Design review of the part shown in the three views and the two pictorial views. Dimensions are in mm from the part's minimum x, y and z. Round coordinates to 2 decimals unless told otherwise and drop trailing zeros. Write each loop counter-clockwise with the first axis right and the second up, starting at its lowest first coordinate (ties: lowest second). Pieces come first, ordered by that corner, then holes. Notation, with made-up numbers: (63, 71) - (70, 71) arc R21 ccw to (70, 87) - close; hole circle Ø11 at (58.5, 71). An arc over 180 degrees is marked (long way). One line per item, written item: value. Start each with the question number.
Q1. Add section D-D on y = 37.5. Write out the cut boundary in (x, z), and give its area (3 significant figures).
Q2. For probe 1 along Z at (x, y) = (15.5, 21); probe 2 along X at (y, z) = (3, 3.5), list the stretches that pass through material, from the lowest coordinate up.
Q3. Add section B-B on x = 27.5. Write out the cut boundary in (y, z), and give its area (3 significant figures).
Q4. Add section A-A on y = 22. Write out the cut boundary in (x, z), and give its area (3 significant figures).
Q5. Mouldability with a two-part tool opening along Z and no side actions: class the marked faces 1, 2 and 3 as +Z half, -Z half, draft (parallel to the pull), parting line (faces both ways), or undercut.
Q6. Add section C-C on x = 17. Write out the cut boundary in (y, z), and give its area (3 significant figures).
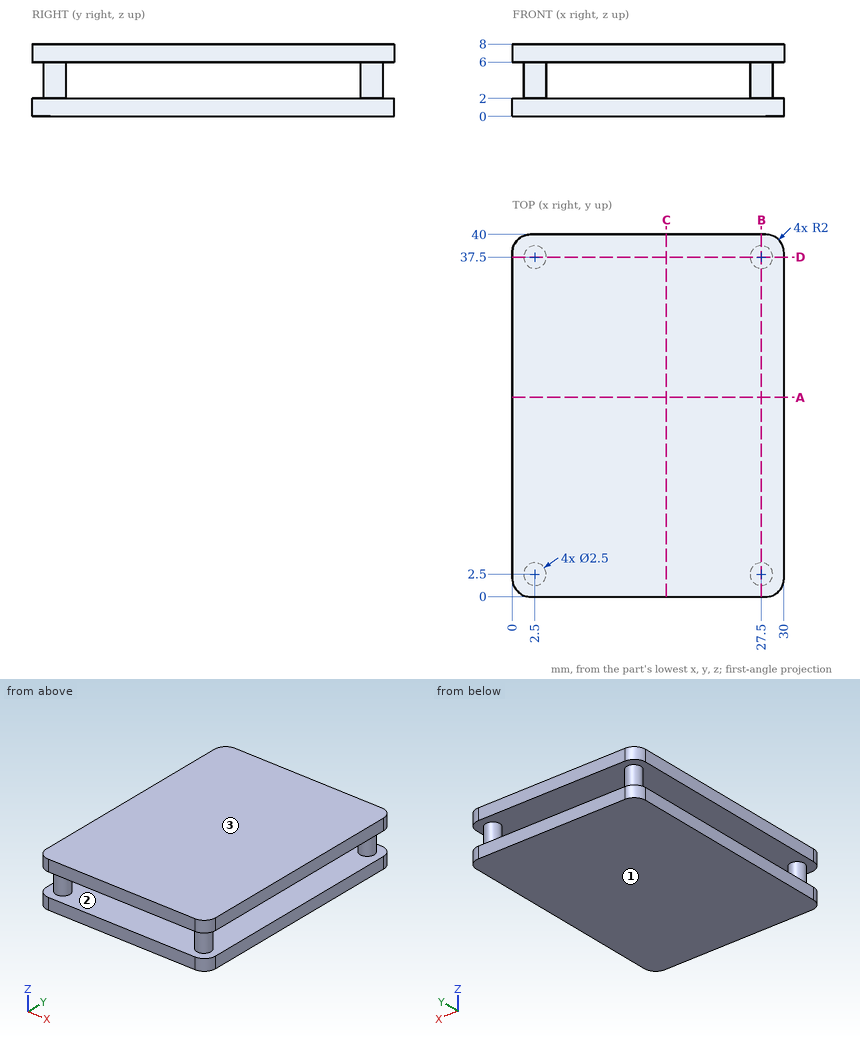
Result set:
1. outline: (0, 0) - (30, 0) - (30, 2) - (28.75, 2) - (28.75, 6) - (30, 6) - (30, 8) - (0, 8) - (0, 6) - (1.25, 6) - (1.25, 2) - (0, 2) - close; hole (3.75, 2) - (26.25, 2) - (26.25, 6) - (3.75, 6) - close
1. area: 140 mm^2
2. probe 1: z = 0 to 2, 6 to 8
2. probe 2: x = 1.35 to 3.65, 26.35 to 28.65
3. outline: (0, 0) - (40, 0) - (40, 2) - (38.75, 2) - (38.75, 6) - (40, 6) - (40, 8) - (0, 8) - (0, 6) - (1.25, 6) - (1.25, 2) - (0, 2) - close; hole (3.75, 2) - (36.25, 2) - (36.25, 6) - (3.75, 6) - close
3. area: 180 mm^2
4. outline: (0, 0) - (30, 0) - (30, 2) - (0, 2) - close; (0, 6) - (30, 6) - (30, 8) - (0, 8) - close
4. area: 120 mm^2
5. face 1: -Z half
5. face 2: undercut
5. face 3: +Z half
6. outline: (0, 0) - (40, 0) - (40, 2) - (0, 2) - close; (0, 6) - (40, 6) - (40, 8) - (0, 8) - close
6. area: 160 mm^2
